from build123d import *

# Parameters (mm, degrees)
F_1_FR_W        = 162.591921451
F_1_FR_H        = 106.952100423
F_1_FR_R        = 3.052899236
EXTRUDE_1_DEPTH = 10


with BuildPart() as part:
    # Эскиз1_fr → Бобышка-Вытянуть1 (new body)
    with BuildSketch(Plane.XY):
        with Locations((41.575310714, -4.636651753)):
            Rectangle(F_1_FR_W, F_1_FR_H)
        with Locations((-22.101373353, 38.438130748)):
            Circle(F_1_FR_R, mode=Mode.SUBTRACT)
        with Locations((5.621100062, 34.197733999)):
            Circle(F_1_FR_R, mode=Mode.SUBTRACT)
        with Locations((33.343573478, 29.95733725)):
            Circle(F_1_FR_R, mode=Mode.SUBTRACT)
        with Locations((61.066046893, 25.716940501)):
            Circle(F_1_FR_R, mode=Mode.SUBTRACT)
        with Locations((5.621100062, 4.197733999)):
            Circle(F_1_FR_R, mode=Mode.SUBTRACT)
        with Locations((33.343573478, -0.04266275)):
            Circle(F_1_FR_R, mode=Mode.SUBTRACT)
        with Locations((61.066046893, -4.283059499)):
            Circle(F_1_FR_R, mode=Mode.SUBTRACT)
        with Locations((5.621100062, -25.802266001)):
            Circle(F_1_FR_R, mode=Mode.SUBTRACT)
        with Locations((33.343573478, -30.04266275)):
            Circle(F_1_FR_R, mode=Mode.SUBTRACT)
        with Locations((61.066046893, -34.283059499)):
            Circle(F_1_FR_R, mode=Mode.SUBTRACT)
        with Locations((-22.101373353, 8.438130748)):
            Circle(F_1_FR_R, mode=Mode.SUBTRACT)
        with Locations((-22.101373353, -21.561869252)):
            Circle(F_1_FR_R, mode=Mode.SUBTRACT)
        with BuildLine():
            ThreePointArc((-26.934111294, 47.298150306), (-32.191806267, 38.242002753), (-26.586166309, 29.39700611))
            ThreePointArc((-26.586166309, 29.39700611), (-23.441936327, 30.456169349), (-24.501099566, 33.60039933))
            ThreePointArc((-24.501099566, 33.60039933), (-27.500569391, 38.33318644), (-24.687278216, 43.178956331))
            ThreePointArc((-24.687278216, 43.178956331), (-23.751097767, 46.361969857), (-26.934111294, 47.298150306))
        make_face(mode=Mode.SUBTRACT)
        with BuildLine():
            ThreePointArc((0.788362122, 43.057753557), (-4.469332851, 34.001606003), (1.136307107, 25.156609361))
            ThreePointArc((1.136307107, 25.156609361), (4.280537088, 26.2157726), (3.22137385, 29.360002581))
            ThreePointArc((3.22137385, 29.360002581), (0.221904024, 34.092789691), (3.035195199, 38.938559582))
            ThreePointArc((3.035195199, 38.938559582), (3.971375648, 42.121573108), (0.788362122, 43.057753557))
        make_face(mode=Mode.SUBTRACT)
        with BuildLine():
            ThreePointArc((28.510835537, 38.817356808), (23.253140564, 29.761209254), (28.858780522, 20.916212612))
            ThreePointArc((28.858780522, 20.916212612), (32.003010504, 21.975375851), (30.943847265, 25.119605832))
            ThreePointArc((30.943847265, 25.119605832), (27.94437744, 29.852392942), (30.757668615, 34.698162832))
            ThreePointArc((30.757668615, 34.698162832), (31.693849064, 37.881176359), (28.510835537, 38.817356808))
        make_face(mode=Mode.SUBTRACT)
        with BuildLine():
            ThreePointArc((56.233308952, 34.576960059), (50.97561398, 25.520812505), (56.581253938, 16.675815863))
            ThreePointArc((56.581253938, 16.675815863), (59.725483919, 17.734979101), (58.666320681, 20.879209083))
            ThreePointArc((58.666320681, 20.879209083), (55.666850855, 25.611996193), (58.48014203, 30.457766083))
            ThreePointArc((58.48014203, 30.457766083), (59.416322479, 33.64077961), (56.233308952, 34.576960059))
        make_face(mode=Mode.SUBTRACT)
        with BuildLine():
            ThreePointArc((0.788362122, 13.057753557), (-4.469332851, 4.001606003), (1.136307107, -4.843390639))
            ThreePointArc((1.136307107, -4.843390639), (4.280537088, -3.7842274), (3.22137385, -0.639997419))
            ThreePointArc((3.22137385, -0.639997419), (0.221904024, 4.092789691), (3.035195199, 8.938559582))
            ThreePointArc((3.035195199, 8.938559582), (3.971375648, 12.121573108), (0.788362122, 13.057753557))
        make_face(mode=Mode.SUBTRACT)
        with BuildLine():
            ThreePointArc((28.510835537, 8.817356808), (23.253140564, -0.238790746), (28.858780522, -9.083787388))
            ThreePointArc((28.858780522, -9.083787388), (32.003010504, -8.024624149), (30.943847265, -4.880394168))
            ThreePointArc((30.943847265, -4.880394168), (27.94437744, -0.147607058), (30.757668615, 4.698162832))
            ThreePointArc((30.757668615, 4.698162832), (31.693849064, 7.881176359), (28.510835537, 8.817356808))
        make_face(mode=Mode.SUBTRACT)
        with BuildLine():
            ThreePointArc((56.233308952, 4.576960059), (50.97561398, -4.479187495), (56.581253938, -13.324184137))
            ThreePointArc((56.581253938, -13.324184137), (59.725483919, -12.265020899), (58.666320681, -9.120790917))
            ThreePointArc((58.666320681, -9.120790917), (55.666850855, -4.388003807), (58.48014203, 0.457766083))
            ThreePointArc((58.48014203, 0.457766083), (59.416322479, 3.64077961), (56.233308952, 4.576960059))
        make_face(mode=Mode.SUBTRACT)
        with BuildLine():
            ThreePointArc((0.788362122, -16.942246443), (-4.469332851, -25.998393997), (1.136307107, -34.843390639))
            ThreePointArc((1.136307107, -34.843390639), (4.280537088, -33.7842274), (3.22137385, -30.639997419))
            ThreePointArc((3.22137385, -30.639997419), (0.221904024, -25.907210309), (3.035195199, -21.061440418))
            ThreePointArc((3.035195199, -21.061440418), (3.971375648, -17.878426892), (0.788362122, -16.942246443))
        make_face(mode=Mode.SUBTRACT)
        with BuildLine():
            ThreePointArc((28.510835537, -21.182643192), (23.253140564, -30.238790746), (28.858780522, -39.083787388))
            ThreePointArc((28.858780522, -39.083787388), (32.003010504, -38.024624149), (30.943847265, -34.880394168))
            ThreePointArc((30.943847265, -34.880394168), (27.94437744, -30.147607058), (30.757668615, -25.301837168))
            ThreePointArc((30.757668615, -25.301837168), (31.693849064, -22.118823641), (28.510835537, -21.182643192))
        make_face(mode=Mode.SUBTRACT)
        with BuildLine():
            ThreePointArc((56.233308952, -25.423039941), (50.97561398, -34.479187495), (56.581253938, -43.324184137))
            ThreePointArc((56.581253938, -43.324184137), (59.725483919, -42.265020899), (58.666320681, -39.120790917))
            ThreePointArc((58.666320681, -39.120790917), (55.666850855, -34.388003807), (58.48014203, -29.542233917))
            ThreePointArc((58.48014203, -29.542233917), (59.416322479, -26.35922039), (56.233308952, -25.423039941))
        make_face(mode=Mode.SUBTRACT)
        with BuildLine():
            ThreePointArc((-26.934111294, 17.298150306), (-32.191806267, 8.242002753), (-26.586166309, -0.60299389))
            ThreePointArc((-26.586166309, -0.60299389), (-23.441936327, 0.456169349), (-24.501099566, 3.60039933))
            ThreePointArc((-24.501099566, 3.60039933), (-27.500569391, 8.33318644), (-24.687278216, 13.178956331))
            ThreePointArc((-24.687278216, 13.178956331), (-23.751097767, 16.361969857), (-26.934111294, 17.298150306))
        make_face(mode=Mode.SUBTRACT)
        with BuildLine():
            ThreePointArc((-26.934111294, -12.701849694), (-32.191806267, -21.757997247), (-26.586166309, -30.60299389))
            ThreePointArc((-26.586166309, -30.60299389), (-23.441936327, -29.543830651), (-24.501099566, -26.39960067))
            ThreePointArc((-24.501099566, -26.39960067), (-27.500569391, -21.66681356), (-24.687278216, -16.821043669))
            ThreePointArc((-24.687278216, -16.821043669), (-23.751097767, -13.638030143), (-26.934111294, -12.701849694))
        make_face(mode=Mode.SUBTRACT)
    extrude(amount=EXTRUDE_1_DEPTH)


solid = part.part
Design review of the part built by this model. Coordinates are the model's own, in mm. A direction names the side the tool comes from. Coordinates: 2 decimals unless noted, no trailing zeros. One line per item, written item: value.
1) Clearance check with flat-ended pins moving along their axes: P1, Ø5.5, axis at x = 33.34, y = 29.96, coming from the +Z side; P2, Ø7, axis at x = 5.62, y = -25.8, coming from the -Z side. State where each tip first meets the part, or that it passes through.
Output values:
P1: passes through
P2: stops at z = 0
2) Draft analysis for pull direction Y (two halves, no side actions). For faces 1 (the face through (-27.5, 38.3, 4.9)), 2 (the face through (40, -4, 10)), state which applies: +Y half, -Y half, draft (parallel to the pull), parting line (faces both ways), or undercut.
Output values:
face 1: undercut
face 2: draft
3) To check wall thickness, follow probe 1 along X at (y, z) = (13, 3.5); probe 2 along X at (y, z) = (10, 8.25); probe 3 along X at (y, z) = (-9, 3.75). State the ranges of each line that lie inside material, in increasing order. Write a range as [from, to].
Output values:
probe 1: x = [-39.72, -31.1], [-24.99, 0.68], [3.14, 122.87]
probe 2: x = [-39.72, -32.07], [-27.27, -24.72], [-19.48, -2.64], [4.03, 122.87]
probe 3: x = [-39.72, 28.69], [31.1, 52.14], [58.44, 122.87]
4) We need section A-A, the plane z = 6. Count the separate pieces of the cut face and the enclosed holes in it, then the cut area to 3 significant figures.
Output values:
separate pieces: 1
enclosed holes: 24
area: 15,900 mm2
5) Machinability: for faces 3 (the face through (122.871, -5, 5)), 4 (the face through (-4.47, 4.16, 4.93)), which of the approach directions +Z, -Z, +X, -X, +Y, -Y give a long, thin tool a straight path to every point of the face, cutting with its end or side? Answer none if there is none.
Output values:
face 3: +Z, -Z, +X, +Y, -Y
face 4: +Z, -Z
